```python
from build123d import *

# Parameters (mm, degrees)
F0_W      = 77.216
F0_H      = 57.023
F1_DEPTH  = 101.3714
F4_DEPTH  = 101.3724
F6_R      = 6.35
F7_DEPTH  = 57.024
F8_R      = 15.24
F9_DEPTH  = 23.0632
F10_R     = 20.574
F11_DEPTH = 12.7
F12_W     = 54.8132
F12_H     = 2.54
F13_DEPTH = 12.7
F14_SIZE  = 5.08
F15_R     = 5.08
F16_R     = 2.54
F18_DEPTH = 26.036
F19_R     = 1.4224
F20_DEPTH = 64.135
F19_R_2   = 1.905
F21_DEPTH = 45.466
F19_R_3   = 3.5052
F22_DEPTH = 39.116
F23_R     = 1.4732
F23_R_2   = 1.7272
F24_DEPTH = 12.7
F25_R     = 1.4732
F25_R_2   = 1.7272
F26_DEPTH = 12.7
F26_TAPER = -3


with BuildPart() as f1:
    # F0 (on Front) → F1 (new body)
    with BuildSketch(Plane.XZ):
        Rectangle(F0_W, F0_H)
    extrude(amount=F1_DEPTH)

    # F3 (on face) → F4 (cut, through all)
    with BuildSketch(Plane.XZ.offset(101.3714)):
        Polygon((35.306, -28.5115), (38.608, -28.5115), (38.608, 15.8115), (-24.7396, 15.8115), (-24.7396, -2.4765), (9.652, -2.4765), (9.652, -25.5397), (35.306, -25.5397), align=None)
    extrude(amount=-F4_DEPTH, mode=Mode.SUBTRACT)

    # F6 (on face) → F7 (cut, through all)
    with BuildSketch(Plane(origin=(0, 0, -28.5115), x_dir=(1, 0, 0), z_dir=(0, 0, -1))):
        with Locations((11.2014, 51.3334)):
            Circle(F6_R)
    extrude(amount=-F7_DEPTH, mode=Mode.SUBTRACT)

    # F8 (on face) → F9 (cut, through all)
    with BuildSketch(Plane.XY.offset(-2.4765)):
        with Locations((11.2014, -51.3334)):
            Circle(F8_R)
    extrude(amount=-F9_DEPTH, mode=Mode.SUBTRACT)

    # F10 (on face) → F11 (cut, through all)
    with BuildSketch(Plane.XY.offset(28.5115)):
        with Locations((11.2014, -51.3334)):
            Circle(F10_R)
    extrude(amount=-F11_DEPTH, mode=Mode.SUBTRACT)

    # F12 (on face) → F13 (cut, through all)
    with BuildSketch(Plane.XY.offset(28.5115)):
        with Locations((11.2014, -51.3334)):
            Rectangle(F12_W, F12_H)
    extrude(amount=-F13_DEPTH, mode=Mode.SUBTRACT)

    # F14
    f14_edges = [f1.edges().sort_by_distance(p)[0] for p in [
        (-38.608, 0, 0),
        (-38.608, -101.3714, 0),
    ]]
    chamfer(f14_edges, length=F14_SIZE)

    # F15
    f15_edges = [f1.edges().sort_by_distance(p)[0] for p in [
        (9.652, -83.932917, -2.4765),
        (9.652, -18.086183, -2.4765),
    ]]
    fillet(f15_edges, radius=F15_R)

    # F16
    f16_edges = [f1.edges().sort_by_distance(p)[0] for p in [
        (38.608, -101.3714, 22.1615),
        (38.608, 0, 22.1615),
        (35.306, -101.3714, -27.0256),
        (35.306, 0, -27.0256),
    ]]
    fillet(f16_edges, radius=F16_R)

    # F17 (on face) → F18 (cut, through all)
    with BuildSketch(Plane(origin=(0, 0, -28.5115), x_dir=(1, 0, 0), z_dir=(0, 0, -1))):
        with BuildLine():
            Line((27.0771505049, 31.5391477372), (32.6644, 34.7649477372))
            ThreePointArc((32.6644, 34.7649477372), (33.1292522628, 36.4998), (31.3944, 36.9646522628))
            Line((31.3944, 36.9646522628), (25.8071505049, 33.7388522628))
            ThreePointArc((25.8071505049, 33.7388522628), (25.3422982421, 32.004), (27.0771505049, 31.5391477372))
        make_face()
        with BuildLine():
            Line((-8.9146494951, 65.5751477372), (-3.3274, 68.8009477372))
            ThreePointArc((-3.3274, 68.8009477372), (-2.8625477372, 70.5358), (-4.5974, 71.0006522628))
            Line((-4.5974, 71.0006522628), (-10.1846494951, 67.7748522628))
            ThreePointArc((-10.1846494951, 67.7748522628), (-10.6495017579, 66.04), (-8.9146494951, 65.5751477372))
        make_face()
    extrude(amount=-F18_DEPTH, mode=Mode.SUBTRACT)

    # F19 (on face) → F20 (cut)
    with BuildSketch(Plane.XZ.offset(101.3714)):
        with Locations((34.163, 22.1615)):
            Circle(F19_R)
    extrude(amount=-F20_DEPTH, mode=Mode.SUBTRACT)

    # F19 (on face) → F21 (cut)
    with BuildSketch(Plane.XZ.offset(101.3714)):
        with Locations((34.163, 22.1615)):
            Circle(F19_R_2)
        with Locations((34.163, 22.1615)):
            Circle(F19_R, mode=Mode.SUBTRACT)
    extrude(amount=-F21_DEPTH, mode=Mode.SUBTRACT)

    # F19 (on face) → F22 (cut)
    with BuildSketch(Plane.XZ.offset(101.3714)):
        with Locations((34.163, 22.1615)):
            Circle(F19_R_3)
        with Locations((34.163, 22.1615)):
            Circle(F19_R_2, mode=Mode.SUBTRACT)
    extrude(amount=-F22_DEPTH, mode=Mode.SUBTRACT)

    # F23 (on face) → F24 (cut, through all)
    with BuildSketch(Plane.XY.offset(28.5115)):
        with Locations((22.5552, -8.5598)):
            Circle(F23_R)
        with Locations((17.6678259177, -26.97218916)):
            Circle(F23_R)
        Polygon((24.8093691796, -12.4430938737), (21.740637653, -11.6285315267), (18.6719061263, -10.8139691796), (15.4136567381, -23.0888952863), (18.4823882648, -23.9034576334), (21.5511197915, -24.7180199804), align=None)
        with Locations((25.2238661051, -29.762910679)):
            Circle(F23_R_2)
    extrude(amount=-F24_DEPTH, mode=Mode.SUBTRACT)

    # F25 (on face) → F26 (cut, through all)
    with BuildSketch(Plane.XY.offset(28.5115)):
        with Locations((-6.6294, -69.6976)):
            Circle(F25_R)
        with Locations((-19.8998323352, -83.3650110803)):
            Circle(F25_R)
        Polygon((-6.5632368758, -74.1872405692), (-8.8411387225, -71.9755018467), (-11.1190405692, -69.7637631242), (-19.9659954594, -78.875370511), (-17.6880936127, -81.0871092336), (-15.410191766, -83.2988479561), align=None)
        with Locations((1.9183511613, -73.9168599248)):
            Circle(F25_R_2)
    extrude(amount=-F26_DEPTH, taper=F26_TAPER, mode=Mode.SUBTRACT)


solid = f1.part
```
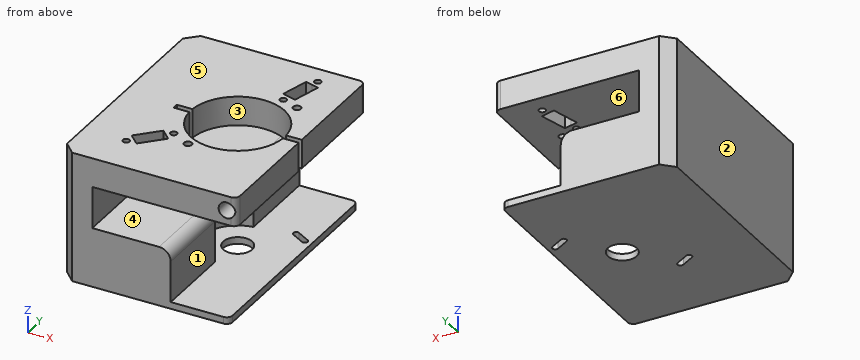
Part model, mm, in its own coordinate system. Face numbers are marked on the shaded views. A direction names the side the tool comes from. Give positions to 0.01 mm unless a question says otherwise; leave off trailing zeros. Loops run counter-clockwise (first coordinate to the right, second up) from the corner with the lowest first, then second, coordinate; pieces in that order, holes last. Notation, with made-up numbers: M 54.5,8.5 L 105.5,8.5 A37 cw 105.5,44.5 Z; hole C 82.25,-30 d8. An arc over 180 degrees is marked long. Return JSON: item names as keys, results as strings.
1) 3-axis set-ups, long thin cutter, end or side, ignore diameter. For the marked faces 5 and 6: which of +Z, -Z, +X, -X, +Y, -Y reach the whole face in a straight line?
Calculated:
{"face 5": "+Z, +X, -X, +Y, -Y", "face 6": "+X, +Y, -Y"}
2) Saw through at A-A, the plane z = -16. List the corners of the cut face in (x, y) (3 decimals).
Calculated:
{"outline": "M -38.608,-96.291 L -33.528,-101.371 L 9.652,-101.371 L 9.652,-66.494 A15.24 cw 9.652,-36.172 L 9.652,0 L -33.528,0 L -38.608,-5.08 Z; hole M -10.185,-67.775 L -4.597,-71.001 A1.27 ccw -3.327,-68.801 L -8.915,-65.575 A1.27 ccw Z"}
3) Flat gauge pins, fed straight in: pin 1 Ø3.5 at (y, z) = (-48.5, -27.5) entering from +X; pin 2 Ø9 at (y, z) = (-88.5, -14) entering from +X; pin 3 Ø1.9 at (x, z) = (33.5, 22) entering from -Y. Where does each tip first touch, or does it go through?
Calculated:
{"pin 1": "stops at x = 35.31", "pin 2": "stops at x = 9.65", "pin 3": "stops at y = -55.91"}
4) Saw through at D-D, the plane y = -91. List the corners of the cut face in (x, z), then the cut area to 3 significant figures.
Calculated:
{"outline": "M -38.61,-28.51 L 35.31,-28.51 L 35.31,-25.54 L 9.65,-25.54 L 9.65,-7.56 A5.08 ccw 4.57,-2.48 L -24.74,-2.48 L -24.74,15.81 L 38.61,15.81 L 38.61,28.51 L -38.61,28.51 Z; hole C 34.16,22.16 d7.01", "area": "2,520 mm2"}
5) Saw through at B-B, the plane y = -39. List the corners of the cut face in (x, z), then the cut area to 3 significant figures.
Calculated:
{"outline": "M -38.61,-28.51 L 35.31,-28.51 L 35.31,-25.54 L 2.25,-25.54 L 2.25,-2.48 L -24.74,-2.48 L -24.74,15.81 L -5.27,15.81 L -5.27,28.51 L -38.61,28.51 Z; M 27.67,15.81 L 38.61,15.81 L 38.61,28.51 L 27.67,28.51 Z; hole C 34.16,22.16 d2.84", "area": "1,970 mm2"}
6) Pull direction X, two halves, no side cores. Call the marked faces 1, 2, 3 and 4: released by +X, released by -X, zero draft, split by the parting line, or undercut.
Calculated:
{"face 1": "released by +X", "face 2": "released by -X", "face 3": "undercut", "face 4": "zero draft"}
7) Saw through at C-C, the plane x = 14. List the corners of the cut face in (y, z).
Calculated:
{"outline": "M -101.37,-28.51 L -57.03,-28.51 L -57.03,-25.54 L -101.37,-25.54 Z; M -101.37,15.81 L -71.72,15.81 L -71.72,28.51 L -101.37,28.51 Z; M -45.63,-28.51 L 0,-28.51 L 0,-25.54 L -45.63,-25.54 Z; M -30.95,15.81 L 0,15.81 L 0,28.51 L -30.95,28.51 Z"}
8) Drill centre lines: line 1 (Z direction, x = -18, y = -73); line 2 (Z direction, x = 35, y = -59); line 3 (Z direction, x = 25, y = -74). Where is each one in solid material? Low to high.
Calculated:
{"line 1": "z = -28.51 to -2.48, 15.81 to 28.51", "line 2": "z = -28.51 to -25.54, 15.81 to 20.45, 23.87 to 28.51", "line 3": "z = -28.51 to -25.54, 15.81 to 28.51"}
